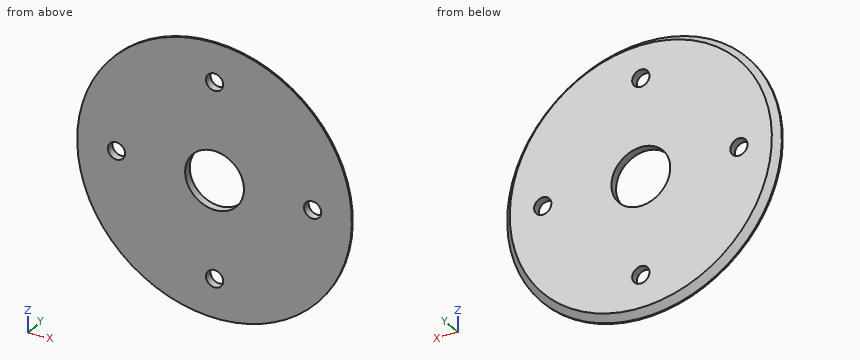
from build123d import *

# Parameters (mm, degrees)
SKETCH1_R           = 35
SKETCH1_R_2         = 2.2
SKETCH1_R_3         = 7.5
BOSS_EXTRUDE1_DEPTH = 2
CHAMFER1_SIZE       = 1.6


with BuildPart() as part:
    # Sketch1 → Boss-Extrude1 (new body)
    with BuildSketch(Plane(origin=(0, 0, 0), x_dir=(1, 0, 0), z_dir=(0, 1, 0))):
        with Locations(Location((0, 0, 0), (0, 0, 270))):
            Circle(SKETCH1_R)
        with Locations(Location((0, 25, 0), (0, 0, 270))):
            Circle(SKETCH1_R_2, mode=Mode.SUBTRACT)
        with Locations(Location((25, 0, 0), (0, 0, 270))):
            Circle(SKETCH1_R_2, mode=Mode.SUBTRACT)
        with Locations(Location((0, -25, 0), (0, 0, 270))):
            Circle(SKETCH1_R_2, mode=Mode.SUBTRACT)
        with Locations(Location((-25, 0, 0), (0, 0, 270))):
            Circle(SKETCH1_R_2, mode=Mode.SUBTRACT)
        with Locations(Location((0, 0, 0), (0, 0, 270))):
            Circle(SKETCH1_R_3, mode=Mode.SUBTRACT)
    extrude(amount=BOSS_EXTRUDE1_DEPTH)

    # Chamfer1
    chamfer1_edges = [part.edges().sort_by_distance(p)[0] for p in [
        (0, 2, -35),
    ]]
    chamfer(chamfer1_edges, length=CHAMFER1_SIZE)


solid = part.part
Verification items for the finished model (mm, model axes). Give positions to 0.01 mm unless a question says otherwise; leave off trailing zeros. Loops run counter-clockwise (first coordinate to the right, second up) from the corner with the lowest first, then second, coordinate; pieces in that order, holes last. Notation, with made-up numbers: (-24, 49.25) - (-2, 49.25) arc R9 ccw to (-2, 58.25) - close; hole circle Ø4 at (-3, -24). An arc over 180 degrees is marked (long way). Write item = value, one per line. Start each with the question number.
Q1. Cross-section at A-A, the plane x = 0. Enter the section's corners in (y, z), and give its area (3 significant figures).
Q2. Thickness scan on line 1 (X direction, y = 0.7, z = 2); line 2 (X direction, y = 1.5, z = 0); line 3 (X direction, y = 1.55, z = -25). Record the ranges inside material, lowest first.
Q3. Cross-section at C-C, the plane y = 0.85. Enter the section's corners in (x, z), and give its area (3 significant figures).
Q4. Cross-section at B-B, the plane z = 0. Enter the section's corners in (x, y).
Q5. Depth check by flat-ended pin: P1, Ø12, axis at x = 0, z = 0, coming from the +Y side. Enter the tip coordinate at first touch or a pass-through.
Answer key:
q1.outline = (0, -35) - (0.4, -35) - (2, -33.4) - (2, -27.2) - (0, -27.2) - close; (0, -22.8) - (2, -22.8) - (2, -7.5) - (0, -7.5) - close; (0, 7.5) - (2, 7.5) - (2, 22.8) - (0, 22.8) - close; (0, 27.2) - (2, 27.2) - (2, 33.4) - (0.4, 35) - (0, 35) - close
q1.area = 89.8 mm^2
q2.line_1 = -34.64 to -25.92, -24.08 to -7.23, 7.23 to 24.08, 25.92 to 34.64
q2.line_2 = -33.9 to -27.2, -22.8 to -7.5, 7.5 to 22.8, 27.2 to 33.9
q2.line_3 = -22.82 to -2.2, 2.2 to 22.82
q3.outline = circle Ø69.1 at (0, 0); hole circle Ø4.4 at (-25, 0); hole circle Ø15 at (0, 0); hole circle Ø4.4 at (0, -25); hole circle Ø4.4 at (0, 25); hole circle Ø4.4 at (25, 0)
q3.area = 3,510 mm^2
q4.outline = (-35, 0) - (-27.2, 0) - (-27.2, 2) - (-33.4, 2) - (-35, 0.4) - close; (-22.8, 0) - (-7.5, 0) - (-7.5, 2) - (-22.8, 2) - close; (7.5, 0) - (22.8, 0) - (22.8, 2) - (7.5, 2) - close; (27.2, 0) - (35, 0) - (35, 0.4) - (33.4, 2) - (27.2, 2) - close
q5.P1 = through
